from build123d import *

# Parameters (mm, degrees)
F1_DEPTH = 20
F2_DEPTH = 10


with BuildPart() as f1:
    # F0 (on Front) → F1 (new body, symmetric)
    with BuildSketch(Plane.XZ):
        Polygon((0, 60), (0, 0), (60, 0), (60, 20), (40, 20), (20, 20), (20, 40), (20, 60), align=None)
    extrude(amount=F1_DEPTH, both=True)

    # F0 (on Front) → F2 (join, symmetric)
    with BuildSketch(Plane.XZ):
        Polygon((0, 60), (0, 0), (60, 0), (60, 20), (40, 20), (20, 20), (20, 40), (20, 60), align=None)
        Polygon((60, 60), (20, 60), (20, 40), (40, 40), (40, 20), (60, 20), align=None)
    extrude(amount=F2_DEPTH, both=True)


solid = f1.part
Could you check a few things on this model? Use its own coordinates, in mm. A direction names the side the tool comes from. Coordinates: 2 decimals unless noted, no trailing zeros. Write each loop counter-clockwise with the first axis right and the second up, starting at its lowest first coordinate (ties: lowest second). Pieces come first, ordered by that corner, then holes. Notation, with made-up numbers: (35.25, 45) - (83.25, 45) arc R34 cw to (83.25, 83) - close; hole circle Ø11 at (-34.5, 58.25). An arc over 180 degrees is marked (long way). Put each result on its own line as item: value. Start each with the question number.
Q1. Thinking about a two-plate mould opening in Z: for faces 6 (the flat face through (30, 0, 0)), 7 (the flat face through (0, 0, 30)), 8 (the flat face through (24, 0, 60)), 9 (the flat face through (36, 0, 20)), which applies, pulls with the +Z half, pulls with the -Z half, needs draft (parallel to the pull), parting line crosses it, or undercut?
Q2. I want a section at A-A on z = 24. Write out the boundary of the cut face in (x, y), plus the area to 3 significant figures.
Q3. I want a section at C-C on y = -1.5. Write out the boundary of the cut face in (x, z), plus the area to 3 significant figures.
Q4. I want a section at B-B on x = 34.5. Write out the boundary of the cut face in (y, z).
Q5. Which directions (+Z, -Z, +X, -X, +Y, -Y) give clear straight access to the entire face, cutting with the end or side of a thin tool? Please do faces 1 (the flat face through (44, -10, 45)), 2 (the flat face through (60, 0, 23)), 3 (the flat face through (40, 0, 30)), 4 (the flat face through (20, 0, 35)), 5 (the flat face through (44, 10, 45)).
Q6. Please list where these lines run through material, in increasing order: L1, parallel to X at y = -6.5, z = 24.5; L2, parallel to Z at x = 23.5, y = -12.
Q7. I want a section at D-D on z = 47. Write out the boundary of the cut face in (x, y).
Q8. I'm going to push flat-ended pins straight in: P1, Ø3, axis at y = -14, z = 44, coming from the +X side; P2, Ø12, axis at x = 45, z = 35.5, coming from the +Y side; P3, Ø12, axis at x = 37, z = 38, coming from the -Y side. Where does each tip first touch, or does it pass through?
Checks:
1. face 6: pulls with the -Z half
1. face 7: needs draft
1. face 8: pulls with the +Z half
1. face 9: undercut
2. outline: (0, -20) - (20, -20) - (20, 20) - (0, 20) - close; (40, -10) - (60, -10) - (60, 10) - (40, 10) - close
2. area: 1,200 mm²
3. outline: (0, 0) - (60, 0) - (60, 60) - (0, 60) - close; hole (20, 20) - (40, 20) - (40, 40) - (20, 40) - close
3. area: 3,200 mm²
4. outline: (-20, 0) - (20, 0) - (20, 20) - (-20, 20) - close; (-10, 40) - (10, 40) - (10, 60) - (-10, 60) - close
5. face 1: +Z, +X, -Y
5. face 2: +Z, -Z, +X, +Y, -Y
5. face 3: +Y, -Y
5. face 4: none
5. face 5: +Z, +X, +Y
6. L1: 0 to 20, 40 to 60
6. L2: 0 to 20
7. outline: (0, -20) - (20, -20) - (20, -10) - (60, -10) - (60, 10) - (20, 10) - (20, 20) - (0, 20) - close
8. P1: x = 20
8. P2: y = 10
8. P3: y = -10
